For this review, take the finished solid that the model builds, in its own axes (mm). Round coordinates to 2 decimals unless told otherwise and drop trailing zeros. Loops run counter-clockwise (first coordinate to the right, second up) from the corner with the lowest first, then second, coordinate; pieces in that order, holes last.
1) Take a section at A-A (y = -508). State the section outline as (x, z) points, then the cut area to 3 significant figures.
2) Take a section at C-C (z = -13.5). State the section outline as (x, y) points.
3) Take a section at B-B (x = -44.45). State the section outline as (y, z) points, then the cut area to 3 significant figures.
4) Insertion check: pin 1 (2 mm diameter, centred on x = -15, z = 4, fed in from +Y). The pin has a flat end and moves straight along its axis. Give the tip position at first contact, or say it passes through.
5) Wall thickness on L1, parallel to Y at x = -44.45, z = 9; L2, parallel to Y at x = -44, z = 6; L3, parallel to Y at x = -63, z = 17: over which ranges is each line inside the solid? List them lowest first.
6) Take a section at D-D (x = -76.5). State the section outline as (y, z) points, then the cut area to 3 significant figures.
7) Mouldability with a two-part tool opening along Y and no side actions: class faces 1 (the flat face through (0, -290, 0)), 2 (the flat face through (-45, -546.1, 0)), 3 (the cylindrical face through (-46.103, -495.408, 0.267)) as pulls with the +Y half, pulls with the -Y half, needs draft (parallel to the pull), parting line crosses it, or undercut.
```python
from build123d import *

# Parameters (mm, degrees)
F1_DEPTH = 19.05
F3_DEPTH = 38.101
F4_R     = 12.7
F5_DEPTH = 38.101


with BuildPart() as f1:
    # F0 (on Top) → F1 (new body, symmetric)
    with BuildSketch(Plane.XY):
        Polygon((0, 0), (-88.9, -51.326438931), (-88.9, -546.1), (0, -546.1), align=None)
    extrude(amount=F1_DEPTH, both=True)

    # F2 (on face) → F3 (cut, through all)
    with BuildSketch(Plane.XY.offset(19.05)):
        Polygon((0, -27.5057557238), (0, 0), (-11.9103416036, -6.876438931), align=None)
    extrude(amount=-F3_DEPTH, mode=Mode.SUBTRACT)

    # F4 (on face) → F5 (cut, through all)
    with BuildSketch(Plane.XY.offset(19.05)):
        with Locations((-44.45, -508)):
            Circle(F4_R)
    extrude(amount=-F5_DEPTH, mode=Mode.SUBTRACT)


solid = f1.part
```
Response:
1. outline: (-88.9, -19.05) - (-57.15, -19.05) - (-57.15, 19.05) - (-88.9, 19.05) - close; (-31.75, -19.05) - (0, -19.05) - (0, 19.05) - (-31.75, 19.05) - close
1. area: 2,420 mm2
2. outline: (-88.9, -546.1) - (0, -546.1) - (0, -27.51) - (-11.91, -6.88) - (-88.9, -51.33) - close; hole circle Ø25.4 at (-44.45, -508)
3. outline: (-546.1, -19.05) - (-520.7, -19.05) - (-520.7, 19.05) - (-546.1, 19.05) - close; (-495.3, -19.05) - (-25.66, -19.05) - (-25.66, 19.05) - (-495.3, 19.05) - close
3. area: 18,900 mm2
4. pin 1: stops at y = -8.08
5. L1: y = -546.1 to -520.7, -495.3 to -25.66
5. L2: y = -546.1 to -520.69, -495.31 to -25.4
5. L3: y = -546.1 to -36.37
6. outline: (-546.1, -19.05) - (-44.17, -19.05) - (-44.17, 19.05) - (-546.1, 19.05) - close
6. area: 19,100 mm2
7. face 1: needs draft
7. face 2: pulls with the -Y half
7. face 3: undercut
